Design review of the part built by this model. Coordinates are the model's own, in mm. Face numbers are marked on the shaded views. A direction names the side the tool comes from. Round coordinates to 2 decimals unless told otherwise and drop trailing zeros. Order: outer loops, then holes, each group sorted by start corner. A loop starts at its lowest first (then second) coordinate and runs counter-clockwise, first axis right, second up. Notation, with made-up numbers: (23.25, 71) - (78.25, 71) arc R22 ccw to (78.25, 77) - close; hole circle Ø5 at (-2.75, 41). An arc over 180 degrees is marked (long way). Use CSV: the item, a comma, the result in double quotes.
from build123d import *

# Parameters (mm, degrees)
BOSS_EXTRUDE1_DEPTH = 762


with BuildPart() as part:
    # Sketch2 → Boss-Extrude1 (new body)
    with BuildSketch(Plane.XY):
        with BuildLine():
            Line((-295.882088074, -9.629425512), (-168.882088074, -9.629425512))
            Line((-168.882088074, -9.629425512), (-73.62851045, -9.629425512))
            Line((-73.62851045, -9.629425512), (53.37148955, -9.629425512))
            Line((53.37148955, -9.629425512), (53.37148955, 3.070574488))
            Line((53.37148955, 3.070574488), (-73.62851045, 3.070574488))
            ThreePointArc((-73.62851045, 3.070574488), (-86.550085837, 64.860670535), (-121.255299262, 117.59141338))
            ThreePointArc((-121.255299262, 117.59141338), (-155.960512688, 64.860670535), (-168.882088074, 3.070574488))
            Line((-168.882088074, 3.070574488), (-295.882088074, 3.070574488))
            Line((-295.882088074, 3.070574488), (-295.882088074, -9.629425512))
        make_face()
    extrude(amount=BOSS_EXTRUDE1_DEPTH)


solid = part.part
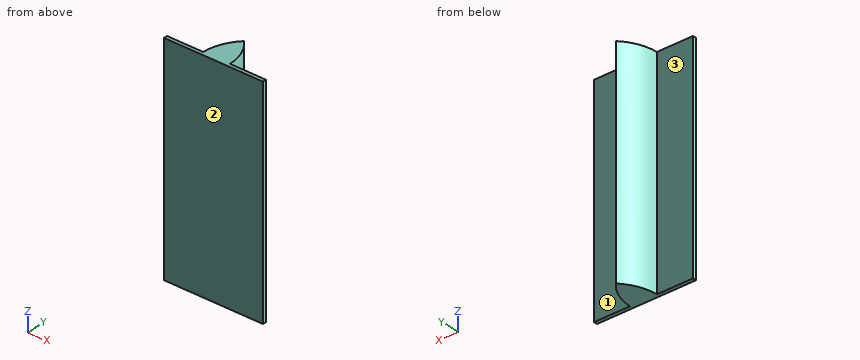
1) Insertion check: pin 1 Ø4 at (y, z) = (94.5, 496) entering from -X; pin 2 Ø1.5 at (y, z) = (20, 293) entering from +X; pin 3 Ø1.5 at (y, z) = (104, 388) entering from -X; pin 4 Ø4 at (x, y) = (-82, 61.5) entering from -Z. Each pin has a flat end and moves straight along its axis. Give the tip position at first contact, or say it passes through.
Data:
pin 1,"stops at x = -141.33"
pin 2,"stops at x = -74.7"
pin 3,"stops at x = -133.68"
pin 4,"passes through"
2) We need section C-C (y = 51.5). Give the boundary of the cut face in (x, z).
Data:
outline,"(-160.87, 0) - (-81.64, 0) - (-81.64, 762) - (-160.87, 762) - close"
3) We need section B-B (x = -55). Give the boundary of the cut face in (y, z), then the cut area to 3 significant figures.
Data:
outline,"(-9.63, 0) - (3.07, 0) - (3.07, 762) - (-9.63, 762) - close"
area,"9,680 mm2"
4) For the marked faces 1, 2 and 3, list the 3-axis set-ups (+Z, -Z, +X, -X, +Y, -Y) from which the entire face can be reached by the end or side of a thin tool; tool diameter is ignored.
Data:
face 1,"+Z, -Z, +X, +Y"
face 2,"+Z, -Z, +X, -X, -Y"
face 3,"+Z, -Z, -X, +Y"
5) We need section A-A (z = 656). Give the boundary of the cut face in (x, y), then the cut area to 3 significant figures.
Data:
outline,"(-295.88, -9.63) - (53.37, -9.63) - (53.37, 3.07) - (-73.63, 3.07) arc R168.91 ccw to (-121.26, 117.59) arc R168.91 ccw to (-168.88, 3.07) - (-295.88, 3.07) - close"
area,"11,900 mm2"
6) To check wall thickness, follow L1, parallel to Y at x = -9.5, z = 346; L2, parallel to X at y = 6.5, z = 577.5; L3, parallel to X at y = 98.5, z = 712.5. State the ranges of each line that lie inside material, in increasing order. Write a range as from..to.
Data:
L1,"y = -9.63..3.07"
L2,"x = -168.78..-73.73"
L3,"x = -137.22..-105.29"
